Here's the drawing with two shaded views (mm, measured from the low corner). I have some questions. Round coordinates to 2 decimals unless told otherwise and drop trailing zeros. Write each loop counter-clockwise with the first axis right and the second up, starting at its lowest first coordinate (ties: lowest second). Pieces come first, ordered by that corner, then holes. Notation, with made-up numbers: M 12.25,31.5 L 28.25,31.5 A20 ccw 28.25,41.5 Z; hole C 86.5,42.25 d9. An arc over 180 degrees is marked long. Use one line per item in the form item = value. Start each with the question number.
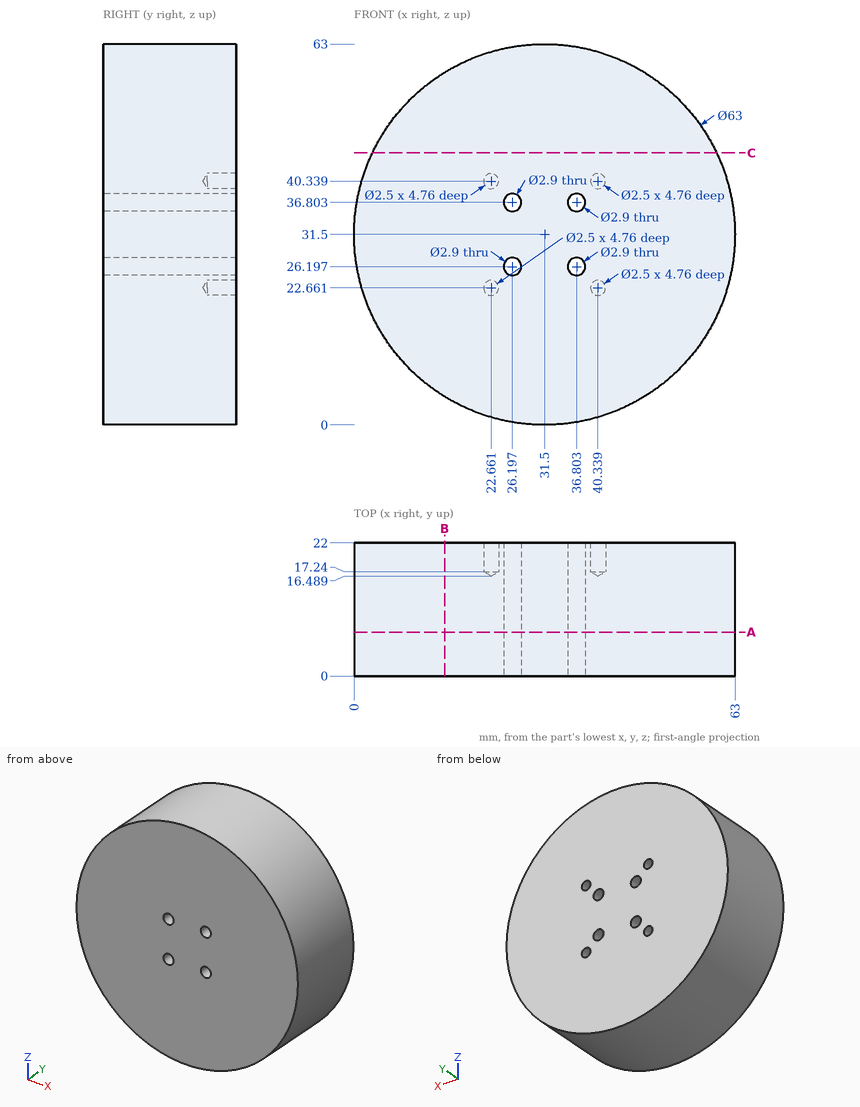
1. If we section it at A-A (y = 7.25): List the corners of the cut face in (x, z) for me.
2. Will these pins go through, and if not, where does the flat tip stop? pin 1 (3 mm diameter, centred on x = 29.5, y = 3, fed in from +Z); pin 2 (1.5 mm diameter, centred on x = 13, y = 17.5, fed in from -Z); pin 3 (5 mm diameter, centred on y = 3, z = 19.5, fed in from -X).
3. Please list where these lines run through material, in increasing order: line 1 along Z through (x, y) = (36.5, 15.75) (1 decimal); line 2 along Z through (x, y) = (26, 1.5); line 3 along X through (y, z) = (13.5, 32.5).
4. If we section it at C-C (z = 45): List the corners of the cut face in (x, y) for me, and give its area (3 significant figures).
5. If we section it at B-B (x = 15): List the corners of the cut face in (y, z) for me.
Model answer:
q1.outline = C 31.5,31.5 d63; hole C 26.2,26.2 d2.9; hole C 26.2,36.8 d2.9; hole C 36.8,26.2 d2.9; hole C 36.8,36.8 d2.9
q2.pin_1 = 63
q2.pin_2 = 5.48
q2.pin_3 = 1.47
q3.line_1 = 0.4 to 24.8, 27.6 to 35.4, 38.2 to 62.6
q3.line_2 = 0.48 to 24.76, 27.63 to 35.37, 38.24 to 62.52
q3.line_3 = 0.02 to 62.98
q4.outline = M 3.04,0 L 59.96,0 L 59.96,22 L 3.04,22 Z
q4.area = 1,250 mm2
q5.outline = M 0,4.67 L 22,4.67 L 22,58.33 L 0,58.33 Z
